Here's how the part is built. I have some questions about the finished solid (model axes, mm). Face numbers are marked on the shaded views. Round coordinates to 2 decimals unless told otherwise and drop trailing zeros. Write each loop counter-clockwise with the first axis right and the second up, starting at its lowest first coordinate (ties: lowest second). Pieces come first, ordered by that corner, then holes. Notation, with made-up numbers: (61.25, -8.75) -> (113.25, -8.75) arc R27 cw to (113.25, 18.25) -> close; hole circle Ø4 at (3, 57.25). An arc over 180 degrees is marked (long way). Answer as CSV lines item,"result".
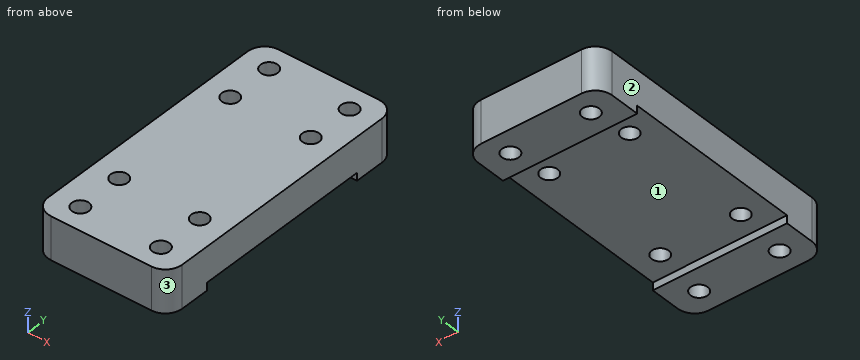
from build123d import *

# Parameters (mm, degrees)
SKETCH1_W           = 40
SKETCH1_H           = 82
SKETCH1_R           = 2.525
BOSS_EXTRUDE1_DEPTH = 12.7
SKETCH2_W           = 40
SKETCH2_H           = 54
CUT_EXTRUDE1_DEPTH  = 2.3
FILLET1_R           = 5


with BuildPart() as part:
    # Sketch1 → Boss-Extrude1 (new body)
    with BuildSketch(Plane.XY):
        Rectangle(SKETCH1_W, SKETCH1_H)
        with Locations((-12, 20)):
            Circle(SKETCH1_R, mode=Mode.SUBTRACT)
        with Locations((-12, 34)):
            Circle(SKETCH1_R, mode=Mode.SUBTRACT)
        with Locations(Location((12, 34, 0), (0, 0, 180))):
            Circle(SKETCH1_R, mode=Mode.SUBTRACT)
        with Locations(Location((12, 20, 0), (0, 0, 180))):
            Circle(SKETCH1_R, mode=Mode.SUBTRACT)
        with Locations((12, -20)):
            Circle(SKETCH1_R, mode=Mode.SUBTRACT)
        with Locations((12, -34)):
            Circle(SKETCH1_R, mode=Mode.SUBTRACT)
        with Locations(Location((-12, -20, 0), (0, 0, 180))):
            Circle(SKETCH1_R, mode=Mode.SUBTRACT)
        with Locations(Location((-12, -34, 0), (0, 0, 180))):
            Circle(SKETCH1_R, mode=Mode.SUBTRACT)
    extrude(amount=BOSS_EXTRUDE1_DEPTH)

    # Sketch2 → Cut-Extrude1 (cut)
    with BuildSketch(Plane(origin=(0, 0, 0), x_dir=(-1, 0, 0), z_dir=(0, 0, -1))):
        Rectangle(SKETCH2_W, SKETCH2_H)
    extrude(amount=-CUT_EXTRUDE1_DEPTH, mode=Mode.SUBTRACT)

    # Fillet1
    fillet1_edges = [part.edges().sort_by_distance(p)[0] for p in [
        (20, -41, 6.35),
        (-20, -41, 6.35),
        (-20, 41, 6.35),
        (20, 41, 6.35),
    ]]
    fillet(fillet1_edges, radius=FILLET1_R)


solid = part.part
Item 1: I need wall thicknesses on L1, parallel to Y at x = 12, z = 7.75 (3 decimals); L2, parallel to X at y = 20, z = 8 (3 decimals); L3, parallel to Y at x = -11, z = 10.5. Which ranges of each line are inside material? Lowest first, please.
Results found:
L1,"y = -41 to -36.525, -31.475 to -22.525, -17.475 to 17.475, 22.525 to 31.475, 36.525 to 41"
L2,"x = -20 to -14.525, -9.475 to 9.475, 14.525 to 20"
L3,"y = -41 to -36.32, -31.68 to -22.32, -17.68 to 17.68, 22.32 to 31.68, 36.32 to 41"
Item 2: If we mould it in two halves opening along Y, with no side actions, what happens to the marked faces 1, 2 and 3? For each: pulls with the +Y half, pulls with the -Y half, needs draft (parallel to the pull), parting line crosses it, or undercut.
Results found:
face 1,"undercut"
face 2,"needs draft"
face 3,"pulls with the -Y half"
Item 3: Suppose I cut it at D-D, the plane y = -20. List the corners of the cut face in (x, z) for me (3 decimals), then the cut area to 3 significant figures.
Results found:
outline,"(-20, 2.3) -> (-14.525, 2.3) -> (-14.525, 12.7) -> (-20, 12.7) -> close; (-9.475, 2.3) -> (9.475, 2.3) -> (9.475, 12.7) -> (-9.475, 12.7) -> close; (14.525, 2.3) -> (20, 2.3) -> (20, 12.7) -> (14.525, 12.7) -> close"
area,"311 mm²"
Item 4: Suppose I cut it at A-A, the plane y = 34. List the corners of the cut face in (x, z) for me (3 decimals), then the cut area to 3 significant figures.
Results found:
outline,"(-20, 0) -> (-14.525, 0) -> (-14.525, 12.7) -> (-20, 12.7) -> close; (-9.475, 0) -> (9.475, 0) -> (9.475, 12.7) -> (-9.475, 12.7) -> close; (14.525, 0) -> (20, 0) -> (20, 12.7) -> (14.525, 12.7) -> close"
area,"380 mm²"
Item 5: Will these pins go through, and if not, where does the flat tip stop? pin 1 (4 mm diameter, centred on x = 12, y = -34, fed in from +Z); pin 2 (6.5 mm diameter, centred on x = 12, y = 20, fed in from -Z).
Results found:
pin 1,"passes through"
pin 2,"stops at z = 2.3"
Item 6: Suppose I cut it at C-C, the plane x = -12. List the corners of the cut face in (y, z) for me (3 decimals), then the cut area to 3 significant figures.
Results found:
outline,"(-41, 0) -> (-36.525, 0) -> (-36.525, 12.7) -> (-41, 12.7) -> close; (-31.475, 0) -> (-27, 0) -> (-27, 2.3) -> (-22.525, 2.3) -> (-22.525, 12.7) -> (-31.475, 12.7) -> close; (-17.475, 2.3) -> (17.475, 2.3) -> (17.475, 12.7) -> (-17.475, 12.7) -> close; (22.525, 2.3) -> (27, 2.3) -> (27, 0) -> (31.475, 0) -> (31.475, 12.7) -> (22.525, 12.7) -> close; (36.525, 0) -> (41, 0) -> (41, 12.7) -> (36.525, 12.7) -> close"
area,"684 mm²"
Item 7: Suppose I cut it at B-B, the plane z = 3.75. State how many separate pieces and enclosed holes the cut face has, then the cut area to 3 significant figures.
Results found:
separate pieces,"1"
enclosed holes,"8"
area,"3,100 mm²"
